Geometry: see drawing. Coordinates: mm, zero at the bounding-box minimum. A direction names the side the tool comes from. Give positions to 0.01 mm unless a question says otherwise; leave off trailing zeros. Loops run counter-clockwise (first coordinate to the right, second up) from the corner with the lowest first, then second, coordinate; pieces in that order, holes last. Notation, with made-up numbers: M 59,4 L 91,4 A24 ccw 91,24 Z; hole C -29.75,62 d7. An arc over 180 degrees is marked long. Return JSON: item names as keys, results as strings. Group by question number.
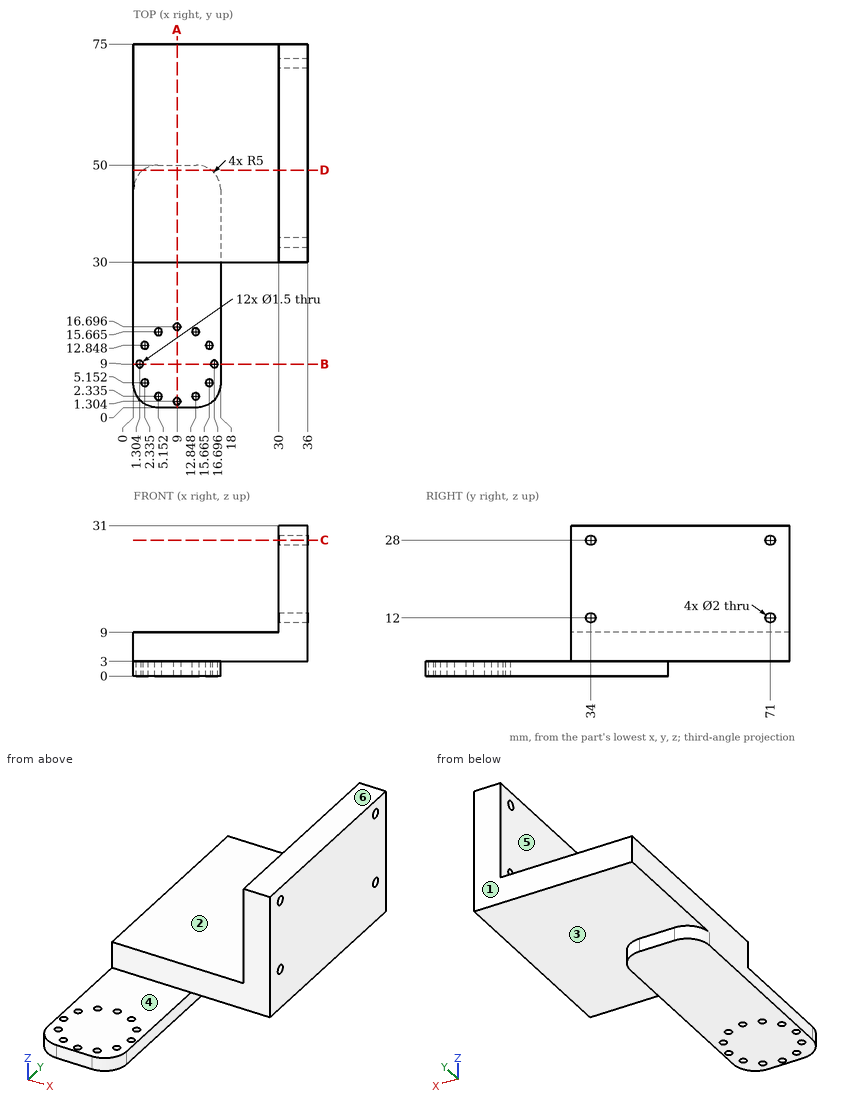
Item 1: First-contact query: pin 1 Ø8 at (y, z) = (39.5, 14) entering from -X; pin 2 Ø1 at (x, z) = (4, 6.5) entering from -Y; pin 3 Ø3.5 at (y, z) = (21, 2) entering from +X. Flat tips, straight axial feed; report the tip coordinate or a pass-through.
Item 2: Section D-D, the plane y = 49. Return loops of the section in (x, z), then the cut area to 3 significant figures.
Item 3: Section B-B, the plane y = 9. Return loops of the section in (x, z).
Item 4: Section C-C, the plane z = 28. Return loops of the section in (x, y).
Item 5: Material intervals for line 1 (Y direction, x = 32.6, z = 12); line 2 (Z direction, x = 33.65, y = 71); line 3 (X direction, y = 9, z = 1), sorted ascending. Write a range as from..to.
Item 6: Reachability of the marked faces 4, 5 and 6 from +Z, -Z, +X, -X, +Y, -Y: full face, straight path, thin tool, end or side. Return the list, or none.
Item 7: Pull-direction query (Z, two-part tool) for the marked faces 1, 2 and 3; classes: pulls with the +Z half, pulls with the -Z half, needs draft (parallel to the pull), parting line crosses it, or undercut.
Item 8: Section A-A, the plane x = 9. Return loops of the section in (y, z), then the cut area to 3 significant figures.
Answer below:
{
 "1": {"pin 1": "x = 30", "pin 2": "y = 30", "pin 3": "x = 18"},
 "2": {"outline": "M 0,3 L 2,3 L 2,0 L 16,0 L 16,3 L 36,3 L 36,31 L 30,31 L 30,9 L 0,9 Z", "area": "390 mm^2"},
 "3": {"outline": "M 0,0 L 0.55,0 L 0.55,3 L 0,3 Z; M 2.05,0 L 15.95,0 L 15.95,3 L 2.05,3 Z; M 17.45,0 L 18,0 L 18,3 L 17.45,3 Z"},
 "4": {"outline": "M 30,30 L 36,30 L 36,33 L 30,33 Z; M 30,35 L 36,35 L 36,70 L 30,70 Z; M 30,72 L 36,72 L 36,75 L 30,75 Z"},
 "5": {"line 1": "30..33, 35..70, 72..75", "line 2": "3..11, 13..27, 29..31", "line 3": "0..0.55, 2.05..15.95, 17.45..18"},
 "6": {"face 4": "+Z, +X, -X, -Y", "face 5": "+Z, -X, +Y, -Y", "face 6": "+Z, +X, -X, +Y, -Y"},
 "7": {"face 1": "needs draft", "face 2": "pulls with the +Z half", "face 3": "pulls with the -Z half"},
 "8": {"outline": "M 0,0 L 0.55,0 L 0.55,3 L 0,3 Z; M 2.05,0 L 15.95,0 L 15.95,3 L 2.05,3 Z; M 17.45,0 L 50,0 L 50,3 L 75,3 L 75,9 L 30,9 L 30,3 L 17.45,3 Z", "area": "411 mm^2"}
}
